Verification items for the finished model (mm, model axes). Face numbers are marked on the shaded views. A direction names the side the tool comes from. Round coordinates to 2 decimals unless told otherwise and drop trailing zeros. Write each loop counter-clockwise with the first axis right and the second up, starting at its lowest first coordinate (ties: lowest second). Pieces come first, ordered by that corner, then holes. Notation, with made-up numbers: (-13, -31.5) -> (17, -31.5) arc R5 ccw to (17, -26.5) -> close; hole circle Ø3 at (-32.75, -18). An arc over 180 degrees is marked (long way). Answer as a JSON object with one key per item and string values. Group by question number.
(1) Sectioned sample at A-A on z = 0. Count the separate pieces of the cut face and the enclosed holes in it, and give its area (3 significant figures).
(2) Gauge pin test, flat ends, axial feed: pin 1 Ø15 at (y, z) = (5, 8.5) entering from +X; pin 2 Ø7.5 at (y, z) = (0, 32.5) entering from -X; pin 3 Ø1.5 at (y, z) = (27.5, 7) entering from -X; pin 4 Ø11.5 at (y, z) = (8, 9) entering from -X. Record the tip position at first contact, or that the pin passes through.
(3) Draft check along Y on the marked faces 1, 2 and 3. Enter one of: released by +Y, released by -Y, zero draft, split by the parting line, or undercut.
(4) Set-up check for the marked faces 4, 5 and 6: record each of +Z, -Z, +X, -X, +Y, -Y from which the full face is reachable in a straight line by a thin tool's end or side.
(5) Sectioned sample at D-D on x = 14.5. Record the cut outline in (y, z), and give its area (3 significant figures).
(6) Scan lines: L1, parallel to Y at x = 12.75, z = 0; L2, parallel to Y at x = -57, z = 0; L3, parallel to X at y = -23, z = 1.5. Record each from-to range of solid material in increasing order. Write a range as from..to.
(7) Sectioned sample at C-C on y = -32.5. Record the cut outline in (x, z), and give its area (3 significant figures).
```python
from build123d import *

# Parameters (mm, degrees)
CHAFL_N1_SIZE         = 3.5
CROQUIS2_R            = 6.25
CORTAR_EXTRUIR2_DEPTH = 27


with BuildPart() as part:
    # Croquis1 → Revolución1 (revolve)
    with BuildSketch(Plane.XY, mode=Mode.PRIVATE) as revoluci_n1_sk:
        Polygon((19.784615385, 15), (-44.615384615, 15), (-44.615384615, 19), (-68.615384615, 19), (-68.615384615, 25), (-38.615384615, 25), (-38.615384615, 20), (5.584615385, 20), (5.584615385, 45), (19.784615385, 45), align=None)
    revolve(revoluci_n1_sk.sketch.rotate(Axis((0, 0, 0), (1, 0, 0)), 90), axis=Axis((0, 0, 0), (1, 0, 0)))

    # Chaflán1
    chafl_n1_edges = [part.edges().sort_by_distance(p)[0] for p in [
        (19.784615385, 0, -15),
    ]]
    chamfer(chafl_n1_edges, length=CHAFL_N1_SIZE)

    # Croquis2 → Cortar-Extruir2 (cut)
    with BuildSketch(Plane.ZY.offset(-5.584615385)):
        with Locations((0, 32.5)):
            Circle(CROQUIS2_R)
        with Locations((0, -32.5)):
            Circle(CROQUIS2_R)
        with Locations((32.5, 0)):
            Circle(CROQUIS2_R)
        with Locations((-32.5, 0)):
            Circle(CROQUIS2_R)
    extrude(amount=-CORTAR_EXTRUIR2_DEPTH, mode=Mode.SUBTRACT)


solid = part.part
```
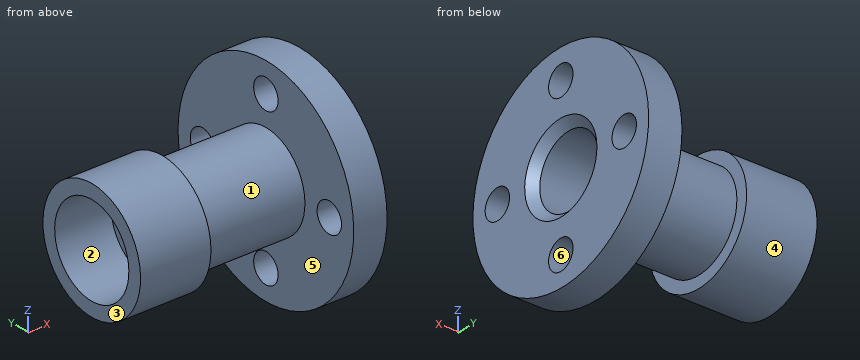
Computed values:
{
 "1": {"separate pieces": "4", "enclosed holes": "0", "area": "1,330 mm2"},
 "2": {"pin 1": "x = 18.65", "pin 2": "through", "pin 3": "x = 5.58", "pin 4": "x = -44.62"},
 "3": {"face 1": "split by the parting line", "face 2": "undercut", "face 3": "zero draft"},
 "4": {"face 4": "-X", "face 5": "none", "face 6": "+X, -X"},
 "5": {"outline": "circle Ø90 at (0, 0); hole circle Ø12.5 at (-32.5, 0); hole circle Ø30 at (0, 0); hole circle Ø12.5 at (0, -32.5); hole circle Ø12.5 at (0, 32.5); hole circle Ø12.5 at (32.5, 0)", "area": "5,160 mm2"},
 "6": {"L1": "-45..-38.75, -26.25..-15, 15..26.25, 38.75..45", "L2": "-25..-19, 19..25", "L3": "-68.62..-38.62, 5.58..19.78"},
 "7": {"outline": "(5.58, -31.12) -> (19.78, -31.12) -> (19.78, -6.25) -> (5.58, -6.25) -> close; (5.58, 6.25) -> (19.78, 6.25) -> (19.78, 31.12) -> (5.58, 31.12) -> close", "area": "706 mm2"}
}
